Autodesk Inventor part; units mm, degrees
ref_plane "YZ Plane" through (0, 0, 0) normal (1, 0, 0) x (0, 1, 0)
ref_plane "XZ Plane" through (0, 0, 0) normal (0, 1, 0) x (-1, 0, 0)
ref_plane "XY Plane" through (0, 0, 0) normal (0, 0, 1) x (1, 0, 0)
sketch "Sketch1" plane through (0, 0, 0) normal (0, 1, 0) x (-1, 0, 0)
  line L0 (-46.4, 46.4) -> (-46.4, -46.4)
  line L1 (-46.4, -46.4) -> (46.4, -46.4)
  line L2 (46.4, -46.4) -> (46.4, 46.4)
  line L3 (46.4, 46.4) -> (-46.4, 46.4)
  line L4 (-46.4, 46.4) -> (46.4, -46.4) construction
  line L5 (-46.4, -46.4) -> (46.4, 46.4) construction
  circle A0 centre (28.15, 0) radius 9.75
  line L6 (-11.62, 56.3044) -> (-11.62, -68.4085) construction
  line L7 (13.88, 18.1678) -> (13.88, -16.702) construction
  line L8 (16.845, 0) -> (-37.12, 0) construction
  line L9 (-37.12, 0) -> (-37.12, -16.702) construction
  line L10 (-37.12, -16.702) -> (-37.12, 16.702) construction
  line L11 (-37.12, 16.702) -> (13.88, 16.702) construction
  line L12 (-37.12, -16.702) -> (13.88, -16.702) construction
  line L13 (13.88, 0) -> (6.92, 0) construction
  circle A1 centre (6.92, 0) radius 4.519 construction
  circle A2 centre (6.92, 0) radius 4.519
  circle A3 centre (-30.16, 0) radius 4.519
  circle A4 centre (-11.62, 0) radius 4.519
  point P0 (0, 0)
  dimension "d0" = 92.8
  dimension "d1" = 92.8
  dimension "d2" = 19.5
  dimension "d3" = 28.15
  dimension "d4" = 11.62
  dimension "d8" = 16.702
  dimension "d9" = 33.404
  dimension "d10" = 6.96
  dimension "d11" = 9.038
  dimension "d46" = 9.038
  dimension "d47" = 6.96
  dimension "d50" = 9.038
extrude "Extrusion1" add sketch "Sketch1" along normal blind 10 contours L3 L2 L1 L0 | A3 | A4
sketch "Sketch2" plane through (0, 10, 0) normal (0, 1, 0) x (1, 0, 0)
  line L0 (-46.4, 46.4) -> (-46.4, -46.4)
  line L1 (46.4, -46.4) -> (46.4, 46.4)
  line L2 (-46.4, -46.4) -> (46.4, 46.4) construction
  line L3 (-46.4, 46.4) -> (46.4, -46.4) construction
  line L4 (-46.4, -44.4) -> (46.4, -44.4) construction
  line L5 (-46.4, 44.4) -> (46.4, 44.4) construction
  line L6 (46.4, 46.4) -> (-46.4, 46.4) construction
  line L7 (-43.9, 46.4) -> (-43.9, -46.4) construction
  line L8 (-46.4, -46.4) -> (46.4, -46.4) construction
  line L9 (43.9, -46.4) -> (43.9, 46.4) construction
  line L10 (-41.4, -42.4) -> (-46.4, -42.4)
  line L11 (-46.4, -42.4) -> (-46.4, -46.4)
  line L12 (-46.4, -46.4) -> (-41.4, -46.4)
  line L13 (-41.4, -46.4) -> (-41.4, -42.4)
  line L14 (-41.4, -42.4) -> (-46.4, -46.4) construction
  line L15 (-46.4, -42.4) -> (-41.4, -46.4) construction
  line L16 (-41.4, 42.4) -> (-46.4, 42.4)
  line L17 (-46.4, 42.4) -> (-46.4, 46.4)
  line L18 (-46.4, 46.4) -> (-41.4, 46.4)
  line L19 (-41.4, 46.4) -> (-41.4, 42.4)
  line L20 (-41.4, 42.4) -> (-46.4, 46.4) construction
  line L21 (-46.4, 42.4) -> (-41.4, 46.4) construction
  line L22 (41.4, 42.4) -> (46.4, 42.4)
  line L23 (46.4, 42.4) -> (46.4, 46.4)
  line L24 (46.4, 46.4) -> (41.4, 46.4)
  line L25 (41.4, 46.4) -> (41.4, 42.4)
  line L26 (41.4, 42.4) -> (46.4, 46.4) construction
  line L27 (46.4, 42.4) -> (41.4, 46.4) construction
  line L28 (41.4, -42.4) -> (46.4, -42.4)
  line L29 (46.4, -42.4) -> (46.4, -46.4)
  line L30 (46.4, -46.4) -> (41.4, -46.4)
  line L31 (41.4, -46.4) -> (41.4, -42.4)
  line L32 (41.4, -42.4) -> (46.4, -46.4) construction
  line L33 (46.4, -42.4) -> (41.4, -46.4) construction
  point P0 (0, 0)
  point P1 (-43.9, -44.4)
  point P2 (-43.9, 44.4)
  point P3 (43.9, 44.4)
  point P4 (43.9, -44.4)
  dimension "d14" = 2.5
  dimension "d15" = 2.5
  dimension "d16" = 2
  dimension "d17" = 2
extrude "Extrusion2" add sketch "Sketch2" along normal blind 3
sketch "Sketch3" plane through (-46.4, 0, 46.4) normal (0, 0, 1) x (1, 0, 0)
  line L0 (0, 10) -> (5, 10) construction
  line L1 (0, 10) -> (92.9772, 10) construction
  line L2 (0, 10) -> (0, 13) construction
  line L3 (5, 10) -> (0, 13) construction
  line L4 (0, 13) -> (5, 13) construction
  line L5 (5, 13) -> (0, 10) construction
  line L6 (92.8, 0) -> (92.8, 13) construction
  line L7 (87.8, 13) -> (92.8, 13) construction
  line L8 (92.8, 10) -> (87.8, 13) construction
  line L9 (87.8, 13) -> (87.8, 10) construction
  line L10 (87.8, 10) -> (92.8, 13) construction
  circle A0 centre (90.3, 11.5) radius 1 construction
  circle A1 centre (90.3, 11.5) radius 1
  circle A2 centre (2.5, 11.5) radius 1
  point P0 (46.4, 0)
  dimension "d20" = 2
  dimension "d21" = 2
sketch "Sketch4" plane through (0, 10, 0) normal (0, 1, 0) x (1, 0, 0)
  line L0 (0, -35.0564) -> (0, -55.3914) construction
  line L1 (-41.4, -46.4) -> (41.4, -46.4)
  line L2 (0, -46.4) -> (-10, -46.4)
  line L3 (-10, -46.4) -> (-10, -38.9)
  line L4 (-10, -38.9) -> (10, -38.9)
  line L5 (10, -38.9) -> (10, -46.4)
  line L6 (0, -46.4) -> (10, -46.4)
  line L7 (-23.157, 0) -> (-56.7416, 0) construction
  line L8 (-56.7416, 0) -> (-56.7416, -46.4) construction
  line L9 (-56.7416, -46.4) -> (-46.4, -46.4) construction
  line L10 (-46.4, -46.4) -> (-56.7416, -23.2) construction
  line L11 (-31.4038, -23.2) -> (-56.7416, -23.2) construction
  line L12 (-46.4, 42.4) -> (-46.4, -42.4)
  line L13 (-46.4, -23.2) -> (-46.4, -33.2)
  line L14 (-46.4, -33.2) -> (-38.9, -33.2)
  line L15 (-38.9, -33.2) -> (-38.9, -13.2)
  line L16 (-38.9, -13.2) -> (-46.4, -13.2)
  line L17 (-46.4, -13.2) -> (-46.4, -23.2)
  line L18 (-50.628, 0) -> (47.2568, 0) construction
  line L19 (0, -71.9527) -> (0, 59.9713) construction
  line L20 (46.4, -23.2) -> (46.4, -33.2)
  line L21 (46.4, -33.2) -> (38.9, -33.2)
  line L22 (38.9, -33.2) -> (38.9, -13.2)
  line L23 (38.9, -13.2) -> (46.4, -13.2)
  line L24 (46.4, -13.2) -> (46.4, -23.2)
  line L25 (0, 46.4) -> (-10, 46.4)
  line L26 (-10, 46.4) -> (-10, 38.9)
  line L27 (-10, 38.9) -> (10, 38.9)
  line L28 (10, 38.9) -> (10, 46.4)
  line L29 (0, 46.4) -> (10, 46.4)
  line L30 (-46.4, 23.2) -> (-46.4, 33.2)
  line L31 (-46.4, 33.2) -> (-38.9, 33.2)
  line L32 (-38.9, 33.2) -> (-38.9, 13.2)
  line L33 (-38.9, 13.2) -> (-46.4, 13.2)
  line L34 (-46.4, 13.2) -> (-46.4, 23.2)
  line L35 (46.4, 33.2) -> (38.9, 33.2)
  line L36 (38.9, 33.2) -> (38.9, 13.2)
  line L37 (38.9, 13.2) -> (46.4, 13.2)
  line L38 (46.4, 13.2) -> (46.4, 23.2)
  line L39 (46.4, 23.2) -> (46.4, 33.2)
  line L40 (9.3, -39.6) -> (-9.3, -39.6) construction
  line L41 (-9.3, -39.6) -> (-9.3, -45.7) construction
  line L42 (-9.3, -45.7) -> (0, -45.7) construction
  line L43 (0, -45.7) -> (9.3, -45.7) construction
  line L44 (9.3, -45.7) -> (9.3, -39.6) construction
  line L45 (-9.3, -39.6) -> (-9.3, -45.7)
  line L46 (-9.3, -45.7) -> (0, -45.7)
  line L47 (0, -45.7) -> (9.3, -45.7)
  line L48 (9.3, -45.7) -> (9.3, -39.6)
  line L49 (9.3, -39.6) -> (-9.3, -39.6)
  line L50 (-39.6, -13.9) -> (-39.6, -32.5)
  line L51 (-39.6, -32.5) -> (-45.7, -32.5)
  line L52 (-45.7, -32.5) -> (-45.7, -23.2)
  line L53 (-45.7, -23.2) -> (-45.7, -13.9)
  line L54 (-45.7, -13.9) -> (-39.6, -13.9)
  line L55 (-45.7, 13.9) -> (-39.6, 13.9)
  line L56 (-39.6, 13.9) -> (-39.6, 32.5)
  line L57 (-39.6, 32.5) -> (-45.7, 32.5)
  line L58 (-45.7, 32.5) -> (-45.7, 23.2)
  line L59 (-45.7, 23.2) -> (-45.7, 13.9)
  line L60 (9.3, 39.6) -> (-9.3, 39.6)
  line L61 (-9.3, 39.6) -> (-9.3, 45.7)
  line L62 (-9.3, 45.7) -> (0, 45.7)
  line L63 (0, 45.7) -> (9.3, 45.7)
  line L64 (9.3, 45.7) -> (9.3, 39.6)
  line L65 (39.6, 13.9) -> (39.6, 32.5)
  line L66 (39.6, 32.5) -> (45.7, 32.5)
  line L67 (45.7, 32.5) -> (45.7, 23.2)
  line L68 (45.7, 23.2) -> (45.7, 13.9)
  line L69 (45.7, 13.9) -> (39.6, 13.9)
  line L70 (39.6, -13.9) -> (39.6, -32.5)
  line L71 (39.6, -32.5) -> (45.7, -32.5)
  line L72 (45.7, -32.5) -> (45.7, -23.2)
  line L73 (45.7, -23.2) -> (45.7, -13.9)
  line L74 (45.7, -13.9) -> (39.6, -13.9)
  point P0 (0, 0)
  dimension "d22" = 10
  dimension "d23" = 7.5
  dimension "d24" = 20
  dimension "d25" = 10
  dimension "d26" = 7.5
  dimension "d27" = 20
  dimension "d28" = 0.7
  dimension "d29" = 0.7
  dimension "d30" = 0.7
  dimension "d31" = 0.7
  dimension "d32" = 0.7
  dimension "d33" = 0.7
  dimension "d34" = 0.7
extrude "Extrusion3" add sketch "Sketch4" along normal blind 10
extrude "Extrusion5" cut sketch "Sketch3" against normal blind 4
ref_plane "Work Plane1" through (46.4, 0, 0) normal (0, 0, -1) x (-1, 0, 0)
mirror "Mirror1" about plane through (46.4, 0, 0) normal (0, 0, -1) of "Extrusion5"
sketch "Sketch6" plane through (0, 10, 0) normal (0, 1, 0) x (1, 0, 0)
  circle A0 centre (-28.15, 0) radius 9.75
  circle A1 centre (-6.92, 0) radius 4.519
  line L0 (10, 46.4) -> (10, 38.9)
  line L1 (10, 38.9) -> (-10, 38.9)
  line L2 (-10, 38.9) -> (-10, 46.4)
  line L3 (-10, 46.4) -> (-41.4, 46.4)
  line L4 (-41.4, 46.4) -> (-41.4, 42.4)
  line L5 (-41.4, 42.4) -> (-46.4, 42.4)
  line L6 (-46.4, 42.4) -> (-46.4, 33.2)
  line L7 (-46.4, 33.2) -> (-38.9, 33.2)
  line L8 (-38.9, 33.2) -> (-38.9, 13.2)
  line L9 (-38.9, 13.2) -> (-46.4, 13.2)
  line L10 (-46.4, 13.2) -> (-46.4, -13.2)
  line L11 (-46.4, -13.2) -> (-38.9, -13.2)
  line L12 (-38.9, -13.2) -> (-38.9, -33.2)
  line L13 (-38.9, -33.2) -> (-46.4, -33.2)
  line L14 (-46.4, -33.2) -> (-46.4, -42.4)
  line L15 (-46.4, -42.4) -> (-41.4, -42.4)
  line L16 (-41.4, -42.4) -> (-41.4, -46.4)
  line L17 (-41.4, -46.4) -> (-10, -46.4)
  line L18 (-10, -46.4) -> (-10, -38.9)
  line L19 (-10, -38.9) -> (10, -38.9)
  line L20 (10, -38.9) -> (10, -46.4)
  line L21 (10, -46.4) -> (41.4, -46.4)
  line L22 (41.4, -46.4) -> (41.4, -42.4)
  line L23 (41.4, -42.4) -> (46.4, -42.4)
  line L24 (46.4, -42.4) -> (46.4, -33.2)
  line L25 (46.4, -33.2) -> (38.9, -33.2)
  line L26 (38.9, -33.2) -> (38.9, -13.2)
  line L27 (38.9, -13.2) -> (46.4, -13.2)
  line L28 (46.4, -13.2) -> (46.4, 13.2)
  line L29 (46.4, 13.2) -> (38.9, 13.2)
  line L30 (38.9, 13.2) -> (38.9, 33.2)
  line L31 (38.9, 33.2) -> (46.4, 33.2)
  line L32 (46.4, 33.2) -> (46.4, 42.4)
  line L33 (46.4, 42.4) -> (41.4, 42.4)
  line L34 (41.4, 42.4) -> (41.4, 46.4)
  line L35 (41.4, 46.4) -> (10, 46.4)
  point P0 (0, 0)
extrude "Extrusion7" add sketch "Sketch6" against normal blind 10 contours A1
extrude "Extrusion9" cut sketch "Sketch1" along normal blind 10 contours A4
sketch "Sketch7" plane through (0, 0, 0) normal (0, -1, 0) x (1, 0, 0)
  line L0 (30.16, 0) -> (30.16, -46.4) construction
  line L1 (41.4, -46.4) -> (10, -46.4)
sketch "Sketch8" plane through (0, 0, 0) normal (0, -1, 0) x (1, 0, 0)
  circle A0 centre (11.62, 0) radius 4.519
  circle A1 centre (-28.15, 0) radius 9.75
  line L0 (46.4, 46.4) -> (46.4, -46.4)
  line L1 (-46.4, 46.4) -> (46.4, 46.4)
  line L2 (-46.4, -46.4) -> (-46.4, 46.4)
  line L3 (46.4, -46.4) -> (-46.4, -46.4)
  circle A2 centre (30.16, 0) radius 4.519
  circle A3 centre (11.62, 0) radius 4.519
  circle A4 centre (-28.15, 0) radius 9.75
  line L4 (46.4, 46.4) -> (46.4, -46.4)
  line L5 (-46.4, 46.4) -> (46.4, 46.4)
  line L6 (-46.4, -46.4) -> (-46.4, 46.4)
  line L7 (46.4, -46.4) -> (-46.4, -46.4)
  line L8 (30.16, 0) -> (30.16, 46.8649) construction
  circle A5 centre (30.16, 30.1599) radius 1.6
  line L9 (55.9453, 0) -> (-55.3311, 0) construction
  line L10 (30.16, 0) -> (30.16, -46.8649) construction
  circle A6 centre (30.16, -30.1599) radius 1.6
  point P0 (0, 0)
  dimension "d53" = 3.2
  dimension "d54" = 30.1599
  dimension "d55" = 30.1599
extrude "Extrusion10" cut sketch "Sketch8" against normal up to surface (10 mm away) contours A5 | A6
properties part number "Lifting Platform With Balance"
Work out the finished part from the listing and answer in its coordinate system (mm). A direction names the side the tool comes from. Round coordinates to 2 decimals unless told otherwise and drop trailing zeros. Write each loop counter-clockwise with the first axis right and the second up, starting at its lowest first coordinate (ties: lowest second). Pieces come first, ordered by that corner, then holes. Notation, with made-up numbers: (-9.5, 57.5) - (46.5, 57.5) arc R17 ccw to (46.5, 66.5) - close; hole circle Ø1 at (59, 12.5). An arc over 180 degrees is marked (long way). Answer in a Markdown table with one row per item. Add a question column.
1. For faces 4 (the flat face through (41.4, 11, -44)), 5 (the cylindrical face through (-44.637, 10.824, -44.428)), 6 (the flat face through (43, 10, 23)), 7 (the flat face through (-43, 15, 13.2)), 8 (the flat face through (39.3, 20, -26.2)), determine the directions among +Z, -Z, +X, -X, +Y, -Y from which every point of the face is accessible in a straight line to the end or side of a thin tool.
2. A cutting plane is placed at C-C, the plane y = 7.75. Determine the outline of the cut face in (x, z), and give its area (3 significant figures).
3. Given pin 1 (4 mm diameter, centred on x = 42, y = 14, fed in from +Z); pin 2 (4 mm diameter, centred on y = 15, z = -41, fed in from +X); pin 3 (3 mm diameter, centred on x = 30.16, z = -30.16, fed in from -Y), each flat-ended and moving along its own axis, determine where each tip first touches the part or whether it passes through.
4. A cutting plane is placed at A-A, the plane x = 30.16. Determine the outline of the cut face in (y, z).
5. The mould has two halves that part along X. Classify faces 1 (the flat face through (-1, 8, 46.4)), 2 (the flat face through (-38.9, 15, -23)), 3 (the flat face through (-39.6, 15, -23)): +X half, -X half, draft (parallel to the pull), parting line (faces both ways), or undercut.
6. Find the intervals of material crossed by line 1 along Z through (x, y) = (30.16, 6.25); line 2 along Z through (x, y) = (9.5, 17.75); line 3 along X through (y, z) = (12.5, -15), in increasing order. Write a range as from..to.
7. A cutting plane is placed at D-D, the plane x = -6.5. Determine the outline of the cut face in (y, z).
8. A cutting plane is placed at B-B, the plane z = 0. Determine the outline of the cut face in (x, y), and give its area (3 significant figures).
Worked out:
| question | item | result |
|---|---|---|
| 1 | face 4 | -Z, +Y |
| 1 | face 5 | -Z |
| 1 | face 6 | +Y |
| 1 | face 7 | +X, -X, +Y |
| 1 | face 8 | +Z, -Z, +X, -X, +Y |
| 2 | outline | (-46.4, -46.4) - (46.4, -46.4) - (46.4, 46.4) - (-46.4, 46.4) - close; hole circle Ø19.5 at (-28.15, 0); hole circle Ø9.04 at (11.62, 0); hole circle Ø3.2 at (30.16, -30.16); hole circle Ø3.2 at (30.16, 30.16) |
| 2 | area | 8,230 mm^2 |
| 3 | pin 1 | z = 46.4 |
| 3 | pin 2 | x = 10 |
| 3 | pin 3 | through |
| 4 | outline | (0, -46.4) - (10, -46.4) - (10, -31.76) - (0, -31.76) - close; (0, -28.56) - (10, -28.56) - (10, 28.56) - (0, 28.56) - close; (0, 31.76) - (10, 31.76) - (10, 46.4) - (0, 46.4) - close |
| 5 | face 1 | draft |
| 5 | face 2 | undercut |
| 5 | face 3 | undercut |
| 6 | line 1 | -46.4..-31.76, -28.56..28.56, 31.76..46.4 |
| 6 | line 2 | -46.4..-38.9, 38.9..46.4 |
| 6 | line 3 | -46.4..-45.7, -39.6..-38.9, 38.9..39.6, 45.7..46.4 |
| 7 | outline | (0, -46.4) - (20, -46.4) - (20, -45.7) - (10, -45.7) - (10, -39.6) - (20, -39.6) - (20, -38.9) - (10, -38.9) - (10, 38.9) - (20, 38.9) - (20, 39.6) - (10, 39.6) - (10, 45.7) - (20, 45.7) - (20, 46.4) - (0, 46.4) - close |
| 8 | outline | (-46.4, 0) - (-37.9, 0) - (-37.9, 10) - (-46.4, 10) - close; (-18.4, 0) - (7.1, 0) - (7.1, 10) - (-18.4, 10) - close; (16.14, 0) - (46.4, 0) - (46.4, 10) - (16.14, 10) - close |
| 8 | area | 643 mm^2 |
